Autodesk Inventor part; units mm, degrees
ref_plane "YZ Plane" through (0, 0, 0) normal (1, 0, 0) x (0, 1, 0)
ref_plane "XZ Plane" through (0, 0, 0) normal (0, 1, 0) x (-1, 0, 0)
ref_plane "XY Plane" through (0, 0, 0) normal (0, 0, 1) x (1, 0, 0)
sketch "Sketch1" plane through (0, 0, 0) normal (0, 0, 1) x (1, 0, 0)
  line L0 (117.4905, 295.341) -> (6.3655, 295.341)
  line L1 (6.3655, 295.341) -> (6.3655, 257.241)
  line L2 (6.3655, 257.241) -> (117.4905, 257.241)
  line L3 (117.4905, 257.241) -> (117.4905, 295.341)
  line L4 (117.4905, 283.403) -> (6.3655, 283.403)
  line L5 (6.3655, 283.403) -> (6.3655, 281.773)
  line L6 (6.3655, 281.773) -> (117.4905, 281.773)
  line L7 (117.4905, 281.773) -> (117.4905, 283.403)
  line L8 (117.4905, 281.773) -> (117.4905, 283.403)
  line L9 (6.3655, 283.403) -> (11.128, 283.403)
  line L10 (11.128, 283.403) -> (11.128, 281.773)
  line L11 (11.128, 281.773) -> (6.3655, 281.773)
  line L12 (6.3655, 281.773) -> (6.3655, 283.403)
  line L13 (117.4905, 283.403) -> (114.3155, 283.403)
  line L14 (114.3155, 283.403) -> (114.3155, 281.773)
  line L15 (114.3155, 281.773) -> (117.4905, 281.773)
  line L16 (117.4905, 281.773) -> (117.4905, 283.403)
  point P0 (0, 0)
  dimension "d0" = 38.1
  dimension "d1" = 111.125
  dimension "d2" = 1.63
  dimension "d3" = 11.938
  dimension "d23" = 103.1875
  dimension "d24" = 3.175
extrude "Extrusion1" add sketch "Sketch1" along normal blind 3.175 contours L3 L4 L1 L0 | L3 L6 L14 L4 | L4 L10 L6 L1 | L3 L2 L1 L6
sketch "Sketch2" plane through (0, 0, 0) normal (0, 0, -1) x (-1, 0, 0)
  line L0 (-114.3155, 283.403) -> (-11.128, 283.403)
  line L1 (-39.7237, 289.3188) -> (-30.1987, 289.3188)
  line L2 (-30.1987, 289.3188) -> (-30.1987, 279.7938)
  line L3 (-30.1987, 279.7938) -> (-39.7237, 279.7938)
  line L4 (-39.7237, 279.7938) -> (-39.7237, 289.3188)
  line L5 (-90.0665, 289.41) -> (-80.5415, 289.41)
  line L6 (-80.5415, 289.41) -> (-80.5415, 279.8923)
  line L7 (-80.5415, 279.8923) -> (-90.0665, 279.8923)
  line L8 (-90.0665, 279.8923) -> (-90.0665, 289.41)
  line L9 (-6.3655, 257.241) -> (-117.4905, 257.241)
  line L10 (-67.3255, 257.241) -> (-44.4655, 257.241)
  line L11 (-117.4905, 295.341) -> (-6.3655, 295.341)
  line L12 (-53.9905, 295.341) -> (-41.2905, 295.341)
  point P0 (0, 0)
  point P1 (-117.4905, 283.403)
  point P2 (-6.3655, 283.403)
  dimension "d8" = 9.525
  dimension "d9" = 9.5177
  dimension "d10" = 9.525
  dimension "d11" = 9.525
  dimension "d13" = 5.9159
extrude "Extrusion2" cut sketch "Sketch2" against normal blind 3.175
properties part number "FrontBulkhead"
The listing builds one solid part. Answer for the finished solid, in the listing's coordinates (mm). A direction names the side the tool comes from. Coordinates: 2 decimals unless noted, no trailing zeros. Loops run counter-clockwise (first coordinate to the right, second up) from the corner with the lowest first, then second, coordinate; pieces in that order, holes last. Notation, with made-up numbers: M 44,45 L 73,45 A5 cw 73,54 Z; hole C -23,79 d6. An arc over 180 degrees is marked long. Answer in a Markdown table with one row per item.
1) Find section A-A (x = 55.5). Determine the outline of the cut face in (y, z) (3 decimals).
Answers below:
| item | result |
|---|---|
| outline | M 257.241,0 L 281.773,0 L 281.773,3.175 L 257.241,3.175 Z; M 283.403,0 L 295.341,0 L 295.341,3.175 L 283.403,3.175 Z |
2) Find the intervals of material crossed by probe 1 along Y at (x, z) = (14, 0.5); probe 2 along X at (y, z) = (286.5, 2.7); probe 3 along Y at (x, z) = (82, 1.5), in increasing order.
Answers below:
| item | result |
|---|---|
| probe 1 | 257.24 to 281.77, 283.4 to 295.34 |
| probe 2 | 6.37 to 30.2, 39.72 to 80.54, 90.07 to 117.49 |
| probe 3 | 257.24 to 279.89, 289.41 to 295.34 |
3) Determine the mould class of faces 3 (the flat face through (90.066, 286, 2)), 4 (the flat face through (61, 277, 3.175)), 5 (the flat face through (117.49, 276, 2)) for opening direction X: released by +X, released by -X, zero draft, split by the parting line, or undercut.
Answers below:
| item | result |
|---|---|
| face 3 | undercut |
| face 4 | zero draft |
| face 5 | released by +X |
4) Find section B-B (z = 2.05). Determine the outline of the cut face in (x, y).
Answers below:
| item | result |
|---|---|
| outline | M 6.37,257.24 L 117.49,257.24 L 117.49,295.34 L 6.37,295.34 Z; hole M 11.13,281.77 L 30.2,281.77 L 30.2,279.79 L 39.72,279.79 L 39.72,281.77 L 80.54,281.77 L 80.54,279.89 L 90.07,279.89 L 90.07,281.77 L 114.32,281.77 L 114.32,283.4 L 90.07,283.4 L 90.07,289.41 L 80.54,289.41 L 80.54,283.4 L 39.72,283.4 L 39.72,289.32 L 30.2,289.32 L 30.2,283.4 L 11.13,283.4 Z |
5) Which of the six approach directions +Z, -Z, +X, -X, +Y, -Y give full straight-line access (tool end or side, diameter ignored) to faces 1 (the flat face through (30.199, 281, 2)), 2 (the flat face through (61, 257.241, 2))?
Answers below:
| item | result |
|---|---|
| face 1 | +Z, -Z |
| face 2 | +Z, -Z, +X, -X, -Y |
